Part print with two shaded views. Sizes in mm from the minimum x, y, z corner. A direction names the side the tool comes from. Coordinates: 2 decimals unless noted, no trailing zeros. Loops run counter-clockwise (first coordinate to the right, second up) from the corner with the lowest first, then second, coordinate; pieces in that order, holes last. Notation, with made-up numbers: M -25.5,-12.75 L -6.5,-12.75 A27 cw -6.5,25.25 Z; hole C 20,-6 d1. An arc over 180 degrees is marked long. Write item = value, one per line. Start each with the question number.
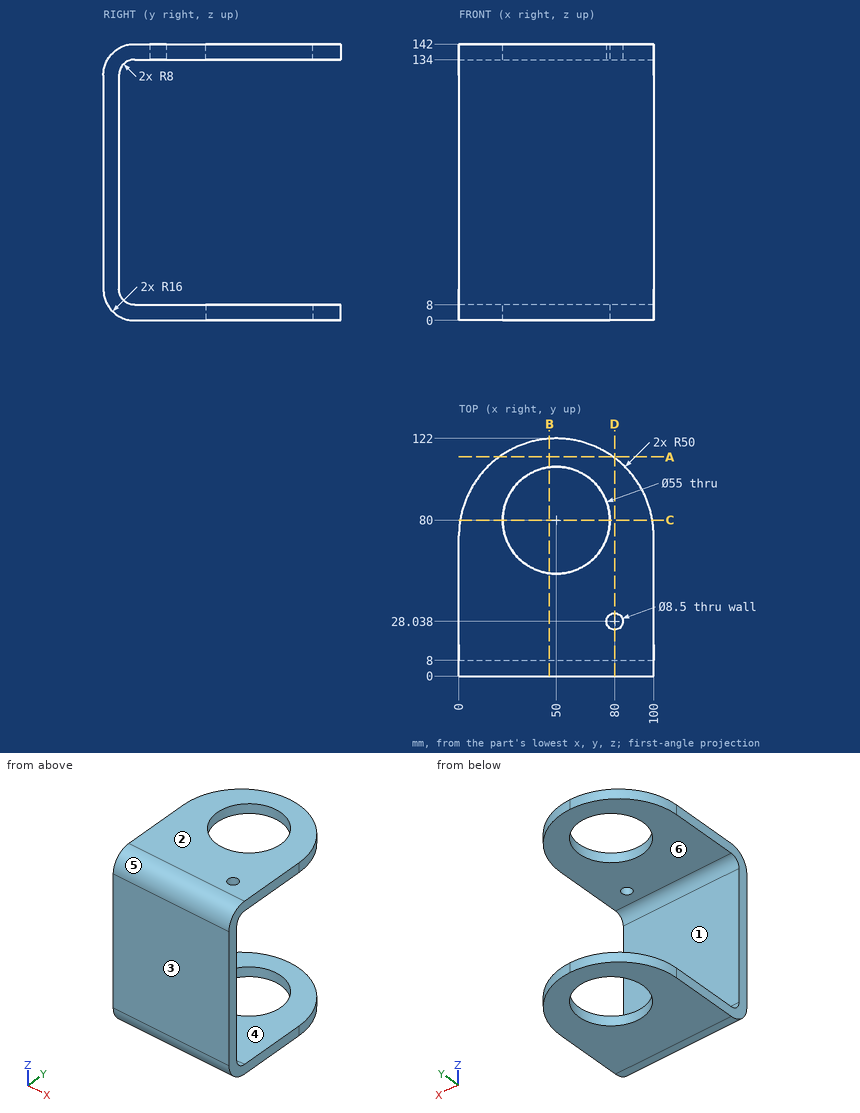
Item 1: 3-axis set-ups, long thin cutter, end or side, ignore diameter. For the marked faces 1 and 2: which of +Z, -Z, +X, -X, +Y, -Y reach the whole face in a straight line?
Item 2: Cut at B-B (x = 46.5). Give the cut face in (y, z), plus the area to 3 significant figures.
Item 3: Probe L1, parallel to Z at x = 89.5, y = 46.5; L2, parallel to Y at x = 93, z = 117.5; L3, parallel to Y at x = 50, z = 3.25 (1 decimal). List the from-to ranges inside material, lowest first.
Item 4: Cut at A-A (y = 112.5). Give the cut face in (x, z).
Item 5: Cut at D-D (x = 80). Give the cut face in (y, z), plus the area to 3 significant figures.
Item 6: Pin check, flat tips, straight feed: pin 1 Ø4 at (x, y) = (63, 13) entering from -Z; pin 2 Ø10 at (x, z) = (32, 20.5) entering from +Y. Stop position of each tip, or through.
Item 7: Cut at C-C (y = 80). Give the cut face in (x, z) (1 decimal).
Item 8: Pull direction Z, two halves, no side cores. Call the marked faces 3, 4, 5 and 6: +Z half, -Z half, draft (parallel to the pull), parting line (faces both ways), or undercut.
Reported:
q1.face_1 = +X, -X, +Y
q1.face_2 = +Z, +X, -X, +Y, -Y
q2.outline = M 0,16 A16 ccw 16,0 L 52.72,0 L 52.72,8 L 16,8 A8 cw 8,16 L 8,126 A8 cw 16,134 L 52.72,134 L 52.72,142 L 16,142 A16 ccw 0,126 Z; M 107.28,0 L 121.88,0 L 121.88,8 L 107.28,8 Z; M 107.28,134 L 121.88,134 L 121.88,142 L 107.28,142 Z
q2.area = 2,000 mm^2
q3.L1 = 0 to 8, 134 to 142
q3.L2 = 0 to 8
q3.L3 = 6.3 to 52.5, 107.5 to 122
q4.outline = M 20.68,0 L 79.32,0 L 79.32,8 L 20.68,8 Z; M 20.68,134 L 79.32,134 L 79.32,142 L 20.68,142 Z
q5.outline = M 0,16 A16 ccw 16,0 L 112,0 L 112,8 L 16,8 A8 cw 8,16 L 8,126 A8 cw 16,134 L 23.79,134 L 23.79,142 L 16,142 A16 ccw 0,126 Z; M 32.29,134 L 112,134 L 112,142 L 32.29,142 Z
q5.area = 2,650 mm^2
q6.pin_1 = 0.03
q6.pin_2 = 8.02
q7.outline = M 0.6,0 L 22.5,0 L 22.5,8 L 0.6,8 Z; M 0.6,134 L 22.5,134 L 22.5,142 L 0.6,142 Z; M 77.5,0 L 99.4,0 L 99.4,8 L 77.5,8 Z; M 77.5,134 L 99.4,134 L 99.4,142 L 77.5,142 Z
q8.face_3 = draft
q8.face_4 = undercut
q8.face_5 = +Z half
q8.face_6 = undercut
